Autodesk Inventor part; units mm, degrees
ref_plane "s1_XY" through (10.3124, 0, 0) normal (0, 0, 1) x (1, 0, 0)
ref_plane "s1_YZ" through (10.3124, 0, 0) normal (1, 0, 0) x (0, 1, 0)
ref_plane "s1_ZX" through (10.3124, 0, 0) normal (0, 1, 0) x (0, 0, 1)
sketch "Sketch_2" plane through (0, 0, 0) normal (0, 0, 1) x (1, 0, 0)
  line L0 (12.7, 0) -> (0, 0)
  line L1 (0, 0) -> (0, 7.098)
  line L2 (0, 7.098) -> (0.8395, 7.9375)
  line L3 (0.8395, 7.9375) -> (6.6816, 7.9375)
  line L4 (6.6816, 7.9375) -> (7.5223, 7.0968)
  arc A0 (7.5223, 7.0968) -> (8.1407, 6.839) centre (8.1385, 7.7041) ccw
  line L5 (8.1407, 6.839) -> (9.4361, 6.839)
  arc A1 (9.4361, 6.839) -> (10.3124, 7.7153) centre (9.4361, 7.7152) ccw
  line L6 (10.3124, 7.7153) -> (10.3124, 7.9057)
  line L7 (10.3124, 7.9057) -> (12.7, 7.9057)
  line L8 (12.7, 7.9057) -> (12.7, 0)
  line L9 (12.7, 0) -> (0, 0)
revolve "Revolution1" add sketch "Sketch_2" angle 360 about axis through (12.7, 0, 0) along (1, 0, 0)
thread "Thread1"
sketch "Sketch_3" plane through (0, 0, 0) normal (0, 0, 1) x (1, 0, 0)
  line L0 (40.4876, 0) -> (12.7, 0)
  line L1 (12.7, 0) -> (12.7, 10.1918)
  line L2 (12.7, 10.1918) -> (13.462, 10.9537)
  line L3 (13.462, 10.9537) -> (34.0741, 10.9537)
  line L4 (34.0741, 10.9537) -> (34.0741, 8.9091)
  line L5 (34.0741, 8.9091) -> (34.8361, 8.9091)
  line L6 (34.8361, 8.9091) -> (35.5981, 9.671)
  line L7 (35.5981, 9.671) -> (39.7256, 9.671)
  line L8 (39.7256, 9.671) -> (40.4876, 8.9091)
  line L9 (40.4876, 8.9091) -> (40.4876, 0)
  line L10 (40.4876, 0) -> (12.7, 0)
revolve "Revolution2" add sketch "Sketch_3" angle 360 about axis through (40.4876, 0, 0) along (1, 0, 0)
sketch "Sketch_5" plane through (0, 0, 0) normal (0, 0, 1) x (1, 0, 0)
  line L0 (40.4876, 0) -> (0, 0)
  line L1 (0, 0) -> (0, 3.4735)
  line L2 (0, 3.4735) -> (0.254, 3.2195)
  line L3 (0.254, 3.2195) -> (40.4876, 3.2195)
  line L4 (40.4876, 3.2195) -> (40.4876, 0)
  line L5 (40.4876, 0) -> (0, 0)
revolve "Revolution3" cut sketch "Sketch_5" angle 360 about axis through (40.4876, 0, 0) along (1, 0, 0)
sketch "Sketch_10" plane through (0, 0, 0) normal (0, 0, 1) x (1, 0, 0)
  line L0 (34.0741, 0) -> (30.8991, 0)
  line L1 (30.8991, 10.2553) -> (34.0741, 10.2553)
  line L2 (34.0741, 10.2553) -> (34.0741, 15.3353)
  line L3 (34.0741, 15.3353) -> (30.8991, 15.3353)
  line L4 (30.8991, 15.3353) -> (30.8991, 10.2553)
revolve "Revolution4" cut sketch "Sketch_10" angle 360 about axis through (34.0741, 0, 0) along (1, 0, 0)
sketch "Sketch_40" plane through (0, 0, 0) normal (0, 1, 0) x (-1, 0, 0)
  line L0 (-24.6126, 10.9537) -> (-24.6126, 0)
  line L1 (-24.6126, 0) -> (-27.7876, 0)
  line L2 (-27.7876, 0) -> (-27.7876, 3.7572)
  line L3 (-27.7876, 3.7572) -> (-29.2538, 4.6037)
  line L4 (-29.2538, 4.6037) -> (-29.4323, 10.3187)
  line L5 (-29.4323, 10.3187) -> (-30.0673, 10.9537)
  line L6 (-30.0673, 10.9537) -> (-24.6126, 10.9537)
  line L7 (-24.6126, 10.9537) -> (-24.6126, 0)
revolve "Revolution5" cut sketch "Sketch_40" angle 360 about axis through (24.6126, 0, 10.9537) along (0, 0, 1)
sketch "Sketch_47" plane through (0, 0, 0) normal (0, 0, 1) x (1, 0, 0)
  line L0 (34.8361, 0) -> (34.0741, 0)
  line L1 (34.0741, 8.655) -> (34.8361, 8.655)
  line L2 (34.8361, 8.655) -> (34.8361, 8.9091)
  line L3 (34.8361, 8.9091) -> (34.4551, 8.9091)
  line L4 (34.4551, 8.9091) -> (34.1966, 9.1676)
  arc A0 (34.1966, 9.3472) -> (34.1966, 9.1676) centre (34.2864, 9.2574) ccw
  line L5 (34.1966, 9.3472) -> (35.0205, 10.1711)
  line L6 (35.0205, 10.1711) -> (35.0205, 10.2553)
  line L7 (35.0205, 10.2553) -> (34.8173, 10.2553)
  line L8 (34.8173, 10.2553) -> (34.0741, 9.512)
  line L9 (34.0741, 9.512) -> (34.0741, 8.655)
revolve "Revolution6" add sketch "Sketch_47" angle 360 about axis through (34.8361, 0, 0) along (1, 0, 0)
ref_plane "s1_XY" through (10.3124, 0, 0) normal (0, 0, 1) x (1, 0, 0)
ref_plane "s1_YZ" through (10.3124, 0, 0) normal (1, 0, 0) x (0, 1, 0)
ref_plane "s1_ZX" through (10.3124, 0, 0) normal (0, 1, 0) x (0, 0, 1)
ref_plane "s2_XY" through (12.7, 0, 0) normal (0, 0, 1) x (1, 0, 0)
ref_plane "s2_YZ" through (12.7, 0, 0) normal (1, 0, 0) x (0, 1, 0)
ref_plane "s2_ZX" through (12.7, 0, 0) normal (0, 1, 0) x (0, 0, 1)
ref_plane "dp1_XY" through (12.7, 7.9057, 0) normal (0, 0, 1) x (1, 0, 0)
ref_plane "dp1_YZ" through (12.7, 7.9057, 0) normal (1, 0, 0) x (0, 1, 0)
ref_plane "dp1_ZX" through (12.7, 7.9057, 0) normal (0, 1, 0) x (0, 0, 1)
ref_plane "dp2_XY" through (12.7, -7.9057, 0) normal (0, 0, 1) x (1, 0, 0)
ref_plane "dp2_YZ" through (12.7, -7.9057, 0) normal (1, 0, 0) x (0, 1, 0)
ref_plane "dp2_ZX" through (12.7, -7.9057, 0) normal (0, 1, 0) x (0, 0, 1)
ref_plane "rod_guide_XY" through (0, 0, 0) normal (1, 0, 0) x (0, 0, -1)
ref_plane "rod_guide_YZ" through (0, 0, 0) normal (0, 0, -1) x (0, 1, 0)
ref_plane "rod_guide_ZX" through (0, 0, 0) normal (0, 1, 0) x (1, 0, 0)
ref_plane "to_tube_XY" through (34.8361, 0, 0) normal (1, 0, 0) x (0, 0, -1)
ref_plane "to_tube_YZ" through (34.8361, 0, 0) normal (0, 0, -1) x (0, 1, 0)
ref_plane "to_tube_ZX" through (34.8361, 0, 0) normal (0, 1, 0) x (1, 0, 0)
ref_plane "to_foot_bracket_XY" through (12.7, 0, 0) normal (1, 0, 0) x (0, 0, -1)
ref_plane "to_foot_bracket_YZ" through (12.7, 0, 0) normal (0, 0, -1) x (0, 1, 0)
ref_plane "to_foot_bracket_ZX" through (12.7, 0, 0) normal (0, 1, 0) x (1, 0, 0)
ref_plane "to_nut_XY" through (10.3124, 0, 0) normal (1, 0, 0) x (0, 0, -1)
ref_plane "to_nut_YZ" through (10.3124, 0, 0) normal (0, 0, -1) x (0, 1, 0)
ref_plane "to_nut_ZX" through (10.3124, 0, 0) normal (0, 1, 0) x (1, 0, 0)
ref_plane "to_trunnion_brackets_XY" through (11.1252, 0, 0) normal (0, 1, 0) x (1, 0, 0)
ref_plane "to_trunnion_brackets_YZ" through (11.1252, 0, 0) normal (1, 0, 0) x (0, 0, -1)
ref_plane "to_trunnion_brackets_ZX" through (11.1252, 0, 0) normal (0, 0, -1) x (0, 1, 0)
ref_plane "to_trunnion_brackets1_XY" through (11.1252, 12.7, 0) normal (0, 1, 0) x (1, 0, 0)
ref_plane "to_trunnion_brackets1_YZ" through (11.1252, 12.7, 0) normal (1, 0, 0) x (0, 0, -1)
ref_plane "to_trunnion_brackets1_ZX" through (11.1252, 12.7, 0) normal (0, 0, -1) x (0, 1, 0)
ref_plane "to_trunnion_brackets2_XY" through (11.1252, -12.7, 0) normal (0, 1, 0) x (1, 0, 0)
ref_plane "to_trunnion_brackets2_YZ" through (11.1252, -12.7, 0) normal (1, 0, 0) x (0, 0, -1)
ref_plane "to_trunnion_brackets2_ZX" through (11.1252, -12.7, 0) normal (0, 0, -1) x (0, 1, 0)
ref_plane "t111_XY" through (12.7, 0, 0) normal (1, 0, 0) x (0, 0, -1)
ref_plane "t111_YZ" through (12.7, 0, 0) normal (0, 0, -1) x (0, 1, 0)
ref_plane "t111_ZX" through (12.7, 0, 0) normal (0, 1, 0) x (1, 0, 0)
ref_plane "t1_XY" through (12.7, 0, 0) normal (1, 0, 0) x (0, 0, -1)
ref_plane "t1_YZ" through (12.7, 0, 0) normal (0, 0, -1) x (0, 1, 0)
ref_plane "t1_ZX" through (12.7, 0, 0) normal (0, 1, 0) x (1, 0, 0)
ref_plane "port_XY" through (24.6126, 0, 0) normal (0, 0, 1) x (1, 0, 0)
ref_plane "port_YZ" through (24.6126, 0, 0) normal (1, 0, 0) x (0, 1, 0)
ref_plane "port_ZX" through (24.6126, 0, 0) normal (0, 1, 0) x (0, 0, 1)
ref_plane "to_screw_XY" through (24.6126, 2.032, -6.0452) normal (0, 1, 0) x (1, 0, 0)
ref_plane "to_screw_YZ" through (24.6126, 2.032, -6.0452) normal (1, 0, 0) x (0, 0, -1)
ref_plane "to_screw_ZX" through (24.6126, 2.032, -6.0452) normal (0, 0, -1) x (0, 1, 0)
properties part number "04R000_rod_guide"
Here's how the part is built. I have some questions about the finished solid (model axes, mm). A direction names the side the tool comes from. Round coordinates to 2 decimals unless told otherwise and drop trailing zeros. Order: outer loops, then holes, each group sorted by start corner. A loop starts at its lowest first (then second) coordinate and runs counter-clockwise, first axis right, second up. Notation, with made-up numbers: M -26.75,32 L 12.25,32 A18 ccw 12.25,54 Z; hole C -3.75,10 d1. An arc over 180 degrees is marked long. Return JSON: item names as keys, results as strings. Group by question number.
1. If we mould it in two halves opening along X, with no side actions, what happens to faces 4 (the face through (30.899, -10, -3)), 5 (the face through (24.2, 3.15, 2.53)), 6 (the face through (32.51, 9.78, 3.08)), 7 (the face through (28.983, -1.812, 7.501))? For each: pulls with the +X half, pulls with the -X half, needs draft (parallel to the pull), parting line crosses it, or undercut.
2. On a 3-axis mill with a long thin cutter (end or side, diameter ignored), from which of +Z, -Z, +X, -X, +Y, -Y can I reach the whole of each face in a straight line? I mean faces 1 (the face through (3.8, -1.72, -7.75)), 2 (the face through (34.648, -1.931, -8.697)), 3 (the face through (22.3, 5.05, -9.72)). Say none if no direction works.
3. If we section it at A-A on x = 36.5: List the corners of the cut face in (y, z) for me, then the cut area to 3 significant figures.
4. Please list where these lines run through material, in increasing order: probe 1 along Z at (x, y) = (14.5, 0); probe 2 along Y at (x, z) = (26.5, -0.25); probe 3 along Z at (x, y) = (21.5, 0).
5. I'm going to push flat-ended pins straight in: pin 1 Ø1 at (x, y) = (4.5, 0.5) entering from -Z; pin 2 Ø10 at (x, z) = (18, -6.5) entering from +Y; pin 3 Ø8.5 at (x, y) = (24.61, 0) entering from +Z. Where does each tip first touch, or does it pass through?
6. If we section it at B-B on y = 0: State how many separate pieces and enclosed holes the cut face has, then the cut area to 3 significant figures.
Reply:
{
 "1": {"face 4": "pulls with the +X half", "face 5": "undercut", "face 6": "needs draft", "face 7": "undercut"},
 "2": {"face 1": "-X", "face 2": "none", "face 3": "+X, -X"},
 "3": {"outline": "C 0,0 d19.34; hole C 0,0 d6.44", "area": "261 mm^2"},
 "4": {"probe 1": "-10.95 to -3.22, 3.22 to 10.95", "probe 2": "-10.95 to -3.21, 3.21 to 10.95", "probe 3": "-10.95 to -3.22"},
 "5": {"pin 1": "z = -7.94", "pin 2": "y = 10.85", "pin 3": "z = 4.38"},
 "6": {"separate pieces": "3", "enclosed holes": "0", "area": "449 mm^2"}
}
